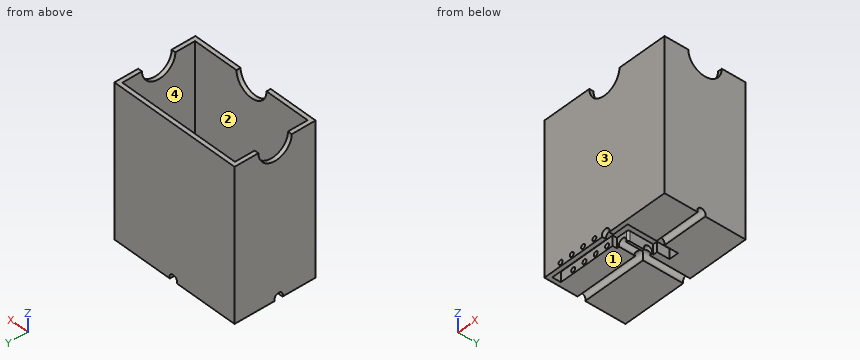
Autodesk Inventor part; units mm, degrees
ref_plane "Work Plane2" through (389.2, 5.1, -50.1) normal (0, 1, 0) x (0, 0, 1)
ref_plane "YZ Plane" through (0, 0, 0) normal (1, 0, 0) x (0, 1, 0)
ref_plane "XZ Plane" through (0, 0, 0) normal (0, 1, 0) x (-1, 0, 0)
sketch "Sketch1" plane through (0, 0, 0) normal (0, 0, 1) x (1, 0, 0)
  line L0 (320.4, 0) -> (420.4, 0) construction
  line L1 (420.4, 0) -> (420.4, -10) construction
  line L2 (320.4, -10) -> (420.4, -10) construction
  line L3 (320.4, 0) -> (320.4, -10) construction
  line L4 (409.3, 0.1) -> (409.3, 50.1) construction
  line L5 (420.4, 0.1) -> (409.3, 0.1) construction
  line L6 (420.4, 50.1) -> (420.4, 0.1) construction
  line L7 (409.3, 50.1) -> (420.4, 50.1) construction
  line L8 (420.5, 50.2) -> (409.2, 50.2)
  line L9 (409.2, 50.2) -> (409.2, 35.3)
  line L10 (409.2, 35.3) -> (404.07, 35.3)
  line L11 (404.07, 35.3) -> (404.07, 7.3)
  line L12 (402.07, 5.3) -> (389.1, 5.3)
  line L13 (389.1, 5.3) -> (389.1, 0.1)
  line L14 (389.1, 0.1) -> (320.3, 0.1)
  line L15 (320.3, 0.1) -> (320.3, -10.1)
  line L16 (320.3, -10.1) -> (420.5, -10.1)
  line L17 (420.5, -10.1) -> (420.5, 50.2)
  arc A0 (402.07, 5.3) -> (404.07, 7.3) centre (402.07, 7.3) ccw
  line L18 (315.3, 5.1) -> (384.1, 5.1)
  line L19 (384.1, 5.1) -> (384.1, 10.3)
  line L20 (384.1, 10.3) -> (399.07, 10.3)
  line L21 (399.07, 10.3) -> (399.07, 40.3)
  line L22 (399.07, 40.3) -> (404.2, 40.3)
  line L23 (404.2, 40.3) -> (404.2, 55.2)
  line L24 (404.2, 55.2) -> (425.5, 55.2)
  line L25 (425.5, 55.2) -> (425.5, -15.1)
  line L26 (425.5, -15.1) -> (315.3, -15.1)
  line L27 (315.3, -15.1) -> (315.3, 5.1)
  line L28 (404.2, 7.2) -> (404.2, 35.2)
  arc A1 (402.2, 5.2) -> (404.2, 7.2) centre (402.2, 7.2) ccw
  line L29 (389.2, 5.2) -> (402.2, 5.2)
  line L30 (389.2, 0.2) -> (389.2, 5.2)
  line L31 (409.2, 0.2) -> (389.2, 0.2)
  line L32 (409.2, 35.2) -> (409.2, 0.2)
  line L33 (404.2, 35.2) -> (409.2, 35.2)
  point P0 (0, 0)
  dimension "d0" = 0.1
  dimension "d1" = 0.1
  dimension "d2" = 0.1
  dimension "d6" = 2
  dimension "d8" = 0.1
  dimension "d9" = 0.1
  dimension "d10" = 0.1
  dimension "d11" = 5
  dimension "d72" = 0.1
  dimension "d73" = 0.1
  dimension "d74" = 0.13
  dimension "d75" = 0.1
extrude "Extrusion1" add sketch "Sketch1" against normal blind 12 contours L18 L19 L20 L21 L22 L23 L24 L25 L26 L27
sketch "Sketch4" plane through (0, 0, 0) normal (0, 0, 1) x (1, 0, 0)
  line L0 (194.6531, 87.1) -> (247.6531, 87.1)
  line L1 (315.3, 82.1) -> (475, 82.1)
  line L2 (475, -15.1) -> (315.3, -15.1)
  line L3 (315.3, -15.1) -> (315.3, 82.1)
  line L4 (315.3, -15.1) -> (425.5, -15.1)
  line L5 (315.3, 5.1) -> (315.3, -15.1)
  line L6 (475, 9.2) -> (475, 65.2)
  line L7 (475, -15.1) -> (475, 82.1)
  point P0 (0, 0)
  dimension "d66" = 5
extrude "Extrusion4" add sketch "Sketch4" along normal blind 169
sketch "Sketch5" plane through (0, 0, 169) normal (0, 0, 1) x (1, 0, 0)
  line L0 (315.3, 82.1) -> (315.3, -15.1)
  line L1 (315.3, -15.1) -> (475, -15.1)
  line L2 (475, -15.1) -> (475, 82.1)
  line L3 (475, 82.1) -> (315.3, 82.1)
  line L4 (320.3, 77.1) -> (320.3, -10.1)
  line L5 (320.3, -10.1) -> (470, -10.1)
  line L6 (470, -10.1) -> (470, 77.1)
  line L7 (470, 77.1) -> (320.3, 77.1)
  point P0 (0, 0)
  dimension "d26" = 5
extrude "Extrusion5" cut sketch "Sketch5" against normal blind 160 contours L7 L6 L5 L4
sketch "Sketch6" plane through (0, 0, 0) normal (0, 0, -1) x (-1, 0, 0)
  line L0 (-384.1, 5.1) -> (-315.3, 5.1)
  line L1 (-315.3, 82.1) -> (-315.3, 5.1)
  line L2 (-475, 82.1) -> (-315.3, 82.1)
  line L3 (-475, -15.1) -> (-475, 82.1)
  line L4 (-425.5, -15.1) -> (-475, -15.1)
  line L5 (-425.5, -15.1) -> (-425.5, 55.2)
  line L6 (-425.5, 55.2) -> (-404.2, 55.2)
  line L7 (-404.2, 55.2) -> (-404.2, 40.3)
  line L8 (-404.2, 40.3) -> (-399.07, 40.3)
  line L9 (-399.07, 40.3) -> (-399.07, 10.3)
  line L10 (-399.07, 10.3) -> (-384.1, 10.3)
  line L11 (-384.1, 10.3) -> (-384.1, 5.1)
  point P0 (0, 0)
extrude "Extrusion6" add sketch "Sketch6" along normal up to surface (12 mm away)
sketch "Sketch7" plane through (315.3, 82.1, 169) normal (0, 1, 0) x (1, 0, 0)
  circle A0 centre (81.4, 179.1) radius 5
  circle A1 centre (36.4, 176.6) radius 2.5 construction
  circle A2 centre (51.4, 176.6) radius 2.5 construction
  circle A3 centre (21.4, 176.6) radius 2.5 construction
  circle A4 centre (66.4, 176.6) radius 2.5 construction
  circle A5 centre (81.4, 179.1) radius 2.5 construction
  circle A6 centre (81.4, 194.1) radius 2.5 construction
  circle A7 centre (81.4, 209.1) radius 2.5 construction
  line L0 (5.1, 169.1) -> (5.1, 312.15) construction
  line L1 (5.1, 312.15) -> (105.1, 312.15) construction
  line L2 (105.1, 312.15) -> (105.1, 169.1) construction
  line L3 (105.1, 169.1) -> (5.1, 169.1) construction
  circle A8 centre (10.1, 282.25) radius 2.15 construction
  circle A9 centre (10.1, 302.15) radius 2.15 construction
  circle A10 centre (88.9, 302.15) radius 2.15 construction
  circle A11 centre (88.9, 282.25) radius 2.15 construction
  circle A12 centre (99.55, 189.1) radius 2.65 construction
  circle A13 centre (99.55, 209.1) radius 2.65 construction
  circle A14 centre (99.55, 229.1) radius 2.65 construction
  circle A15 centre (99.55, 249.1) radius 2.65 construction
  point P0 (-315.3, 169)
  dimension "d71" = 10
ref_plane "Work Plane2" through (389.2, 5.1, -50.1) normal (0, 1, 0) x (0, 0, 1)
extrude "Extrusion7" cut sketch "Sketch7" against normal through all
sketch "Sketch8" plane through (404.07, 7.3, -12) normal (1, 0, 0) x (0, 0, -1)
  circle A0 centre (-1.9, 21.9) radius 2.5 construction
  circle A1 centre (-1.9, 21.9) radius 2.5 construction
  circle A2 centre (-1.9, 21.9) radius 5
  point P0 (-12, -7.3)
  dimension "d34" = 10
extrude "Extrusion8" cut sketch "Sketch8" along normal through all both and the other way through all
sketch "Sketch9" plane through (315.3, -15.1, 169) normal (0, -1, 0) x (1, 0, 0)
  circle A0 centre (81.4, -179.1) radius 3.0567 construction
  line L0 (107.734, -169) -> (7.734, -169) construction
  circle A1 centre (66.4, -176.5) radius 2.65
  circle A2 centre (51.4, -176.5) radius 2.65
  circle A3 centre (36.4, -176.5) radius 2.65
  circle A4 centre (21.4, -176.5) radius 2.65
  line L1 (105.2, -169) -> (5, -169) construction
  circle A5 centre (81.4, -179.1) radius 2.5 construction
  point P0 (-315.3, -169)
  dimension "d37" = 5.3
  dimension "d38" = 7.5
  dimension "d39" = 15
  dimension "d42" = 15
extrude "Extrusion9" cut sketch "Sketch9" against normal blind 45
sketch "Sketch10" plane through (475, -15.1, 169) normal (1, 0, 0) x (0, 0, -1)
  circle A0 centre (0, 48.6) radius 20
  line L0 (0, 48.6) -> (279.056, 48.6) construction
  line L1 (0, 0) -> (0, 97.2)
  point P0 (169, 15.1)
  dimension "d49" = 40
extrude "Extrusion10" cut sketch "Sketch10" against normal through all
fillet "Fillet2" radius 10 4 edges at (395.15, -10.1, 9) (470, 33.5, 9) (395.15, 77.1, 9) (320.3, 33.5, 9)
sketch "Sketch13" plane through (315.3, -15.1, 169) normal (0, -1, 0) x (1, 0, 0)
  line L0 (0, 0) -> (159.7, 0)
  circle A0 centre (79.7, 0) radius 20
  point P0 (-315.3, -169)
  point P1 (99.7, 0)
  point P2 (59.7, 0)
  dimension "d77" = 40
  dimension "d78" = 80
extrude "Extrusion13" cut sketch "Sketch13" against normal up to next contours L0 A0 picked at (83.4871, -5.4866)
properties part number "Lower Support"
For this review, take the finished solid that the model builds, in its own axes (mm). Face numbers are marked on the shaded views. Coordinates: 2 decimals unless noted, no trailing zeros. Loops run counter-clockwise (first coordinate to the right, second up) from the corner with the lowest first, then second, coordinate; pieces in that order, holes last. Notation, with made-up numbers: (13.5, 7.5) - (25.5, 7.5) arc R15 ccw to (25.5, 28.5) - close; hole circle Ø5 at (32.5, -6.5). An arc over 180 degrees is marked (long way). Return JSON: item names as keys, results as strings.
Item 1: Take a section at C-C (y = 18). Give the boundary of the cut face in (x, z), then the cut area to 3 significant figures.
Determined:
{"outline": "(315.3, -12) - (392.08, -12) arc R5 cw (long way) to (401.32, -12) - (404.07, -12) - (404.07, 0) - (420.5, 0) - (420.5, -12) - (475, -12) - (475, 156.36) - (470, 156.36) - (470, 19) arc R10 cw to (460, 9) - (330.3, 9) arc R10 cw to (320.3, 19) - (320.3, 156.36) - (315.3, 156.36) - close; hole circle Ø5.3 at (336.7, -7.5); hole circle Ø5.3 at (351.7, -7.5); hole circle Ø5.3 at (366.7, -7.5); hole circle Ø5.3 at (381.7, -7.5)", "area": "4,530 mm2"}
Item 2: Insertion check: pin 1 (11.5 mm diameter, centred on x = 396.7, z = -10.1, fed in from -Y); pin 2 (12 mm diameter, centred on x = 386, y = 63.5, fed in from +Z); pin 3 (2 mm diameter, centred on x = 346.5, y = -5, fed in from +Z); pin 4 (5 mm diameter, centred on x = 366.7, z = -7.5, fed in from -Y). Each pin has a flat end and moves straight along its axis. Give the tip position at first contact, or say it passes through.
Determined:
{"pin 1": "stops at y = -15.1", "pin 2": "stops at z = 9.29", "pin 3": "stops at z = 10.93", "pin 4": "stops at y = 29.9"}
Item 3: Take a section at A-A (z = 83). Give the boundary of the cut face in (x, y), then the cut area to 3 significant figures.
Determined:
{"outline": "(315.3, -15.1) - (475, -15.1) - (475, 82.1) - (315.3, 82.1) - close; hole (320.3, -10.1) - (470, -10.1) - (470, 77.1) - (320.3, 77.1) - close", "area": "2,470 mm2"}
Item 4: For line 1 (X direction, y = 6, z = 56); line 2 (Y direction, x = 417, z = 57); line 3 (Y direction, x = 463, z = -10.1), list the stretches that pass through material, from the lowest coordinate up.
Determined:
{"line 1": "x = 315.3 to 320.3, 470 to 475", "line 2": "y = -15.1 to -10.1, 77.1 to 82.1", "line 3": "y = -15.1 to 24.2, 34.2 to 82.1"}
Item 5: Mouldability with a two-part tool opening along Y and no side actions: class the marked faces 1, 2, 3 and 4 as pulls with the +Y half, pulls with the -Y half, needs draft (parallel to the pull), parting line crosses it, or undercut.
Determined:
{"face 1": "needs draft", "face 2": "undercut", "face 3": "pulls with the -Y half", "face 4": "undercut"}
Item 6: Take a section at D-D (y = 72). Give the boundary of the cut face in (x, z).
Determined:
{"outline": "(315.3, -12) - (392.08, -12) arc R5 cw (long way) to (401.32, -12) - (475, -12) - (475, 169) - (470, 169) - (470, 19) arc R10 cw to (464.9, 10.28) - (325.4, 10.28) arc R10 cw to (320.3, 19) - (320.3, 169) - (315.3, 169) - close"}
Item 7: Take a section at B-B (x = 455). Give the boundary of the cut face in (y, z).
Determined:
{"outline": "(-15.1, -12) - (24.58, -12) arc R5 cw (long way) to (33.82, -12) - (82.1, -12) - (82.1, 169) - (77.1, 169) - (77.1, 19) arc R10 cw to (67.1, 9) - (-0.1, 9) arc R10 cw to (-10.1, 19) - (-10.1, 169) - (-15.1, 169) - close"}
